Verification items for the finished model (mm, model axes). A direction names the side the tool comes from. Round coordinates to 2 decimals unless told otherwise and drop trailing zeros. Write each loop counter-clockwise with the first axis right and the second up, starting at its lowest first coordinate (ties: lowest second). Pieces come first, ordered by that corner, then holes. Notation, with made-up numbers: M 29.5,-35 L 79.5,-35 A21 cw 79.5,-4 Z; hole C 60,47.25 d9. An arc over 180 degrees is marked long. Answer in a Markdown table with one row per item. Add a question column.
1. Sectioned sample at D-D on x = -91.5. Record the cut outline in (y, z), plus the area to 3 significant figures.
2. Sectioned sample at B-B on x = -80. Record the cut outline in (y, z).
3. Sectioned sample at C-C on y = 0. Record the cut outline in (x, z), plus the area to 3 significant figures.
4. Draft check along Y on faces 3 (the flat face through (-71.855, 12.305, 3.131)), 4 (the cylindrical face through (-95, 15, 3)), 5 (the flat face through (-64, -11, 6.35)). Enter one of: pulls with the +Y half, pulls with the -Y half, needs draft (parallel to the pull), parting line crosses it, or undercut.
5. Material ranges on probe 1 along Y at (x, z) = (-82.5, 4); probe 2 along Y at (x, z) = (-67, 3.25); probe 3 along X at (y, z) = (-9.5, 4.25), recorded low to high.
6. Go/stop test with a flat-tipped pin: pin 1 Ø4 at (x, y) = (-93, -2) entering from -Z. Record where the tip stops, or that it passes through.
7. Set-up check for faces 1 (the flat face through (-87.23, -3.43, 3.13)), 2 (the flat face through (-64, -11, 0)): record each of +Z, -Z, +X, -X, +Y, -Y from which the full face is reachable in a straight line by a thin tool's end or side.
8. Sectioned sample at A-A on z = 5.5. Record the cut outline in (x, y).
Autodesk Inventor part; units mm, degrees
ref_plane "YZ Plane" through (0, 0, 0) normal (1, 0, 0) x (0, 1, 0)
ref_plane "XZ Plane" through (0, 0, 0) normal (0, 1, 0) x (-1, 0, 0)
ref_plane "XY Plane" through (0, 0, 0) normal (0, 0, 1) x (1, 0, 0)
sketch "Sketch1" plane through (0, 0, 0) normal (0, 0, 1) x (1, 0, 0)
  circle A0 centre (-75, 0) radius 25
  circle A1 centre (-75, 0) radius 25
  line L0 (-78.8445, 14.1518) -> (-64.6664, 10.4053)
  line L1 (-64.6664, 10.4053) -> (-60.8219, -3.7465)
  line L2 (-60.8219, -3.7465) -> (-71.1555, -14.1518)
  line L3 (-71.1555, -14.1518) -> (-85.3336, -10.4053)
  line L4 (-85.3336, -10.4053) -> (-89.1781, 3.7465)
  line L5 (-89.1781, 3.7465) -> (-78.8445, 14.1518)
  point P0 (0, 0)
extrude "Extrusion1" add sketch "Sketch1" along normal blind 6.35
properties part number "1-4inch_KnifeSpacer_Piece1"
Geometry check:
| question | item | result |
|---|---|---|
| 1 | outline | M -18.78,0 L 18.78,0 L 18.78,6.35 L -18.78,6.35 Z |
| 1 | area | 239 mm2 |
| 2 | outline | M -24.49,0 L -11.81,0 L -11.81,6.35 L -24.49,6.35 Z; M 12.99,0 L 24.49,0 L 24.49,6.35 L 12.99,6.35 Z |
| 3 | outline | M -100,0 L -88.16,0 L -88.16,6.35 L -100,6.35 Z; M -61.84,0 L -50,0 L -50,6.35 L -61.84,6.35 Z |
| 3 | area | 150 mm2 |
| 4 | face 3 | undercut |
| 4 | face 4 | parting line crosses it |
| 4 | face 5 | needs draft |
| 5 | probe 1 | y = -23.85 to -11.15, 10.47 to 23.85 |
| 5 | probe 2 | y = -23.69 to -9.97, 11.02 to 23.69 |
| 5 | probe 3 | x = -98.12 to -85.58, -66.54 to -51.88 |
| 6 | pin 1 | stops at z = 0 |
| 7 | face 1 | +Z, -Z |
| 7 | face 2 | -Z, +X, -X, +Y, -Y |
| 8 | outline | C -75,0 d50; hole M -89.18,3.75 L -85.33,-10.41 L -71.16,-14.15 L -60.82,-3.75 L -64.67,10.41 L -78.84,14.15 Z |
